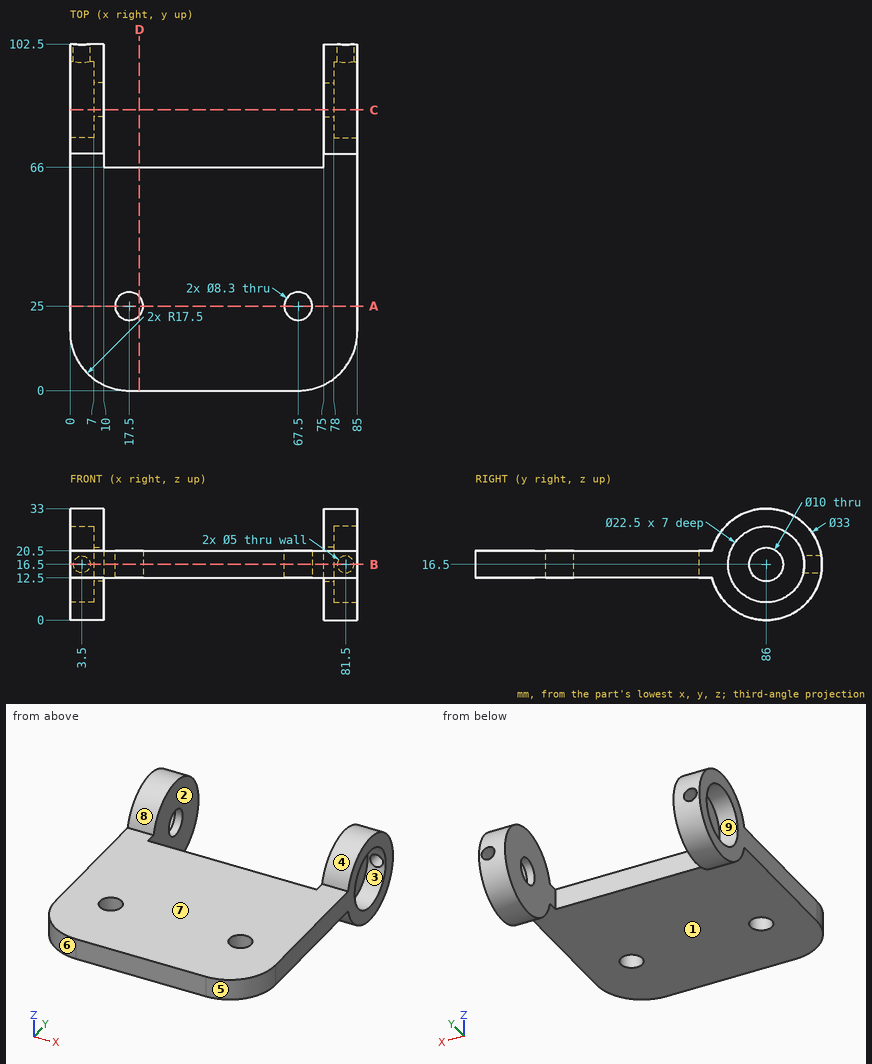
Could you check a few things on this drawing? It's one solid part, dimensions in mm from its lowest x, y, z. A direction names the side the tool comes from. Round coordinates to 2 decimals unless told otherwise and drop trailing zeros. Loops run counter-clockwise (first coordinate to the right, second up) from the corner with the lowest first, then second, coordinate; pieces in that order, holes last. Notation, with made-up numbers: M 31,-30.75 L 42,-30.75 A23 ccw 42,7.25 Z; hole C 12,48 d11. An arc over 180 degrees is marked long. Write each question's results on one line, items separated by ' | '. Start each with the question number.
(1) I want a section at D-D (x = 20.5). Please give me the cut outline in (y, z).
(2) I want a section at C-C (y = 83). Please give me the cut outline in (x, z).
(3) I want a section at B-B (z = 16.5). State how many separate pieces and enclosed holes the cut face has, then the cut area to 3 significant figures.
(4) Will these pins go through, and if not, where does the flat tip stop? P1, Ø3, axis at x = 59.5, z = 11.5, coming from the +Y side; P2, Ø16, axis at y = 86, z = 16.5, coming from the +X side; P3, Ø12, axis at x = 21, z = 28.5, coming from the +Y side; P4, Ø18, axis at y = 86, z = 16, coming from the -X side.
(5) On a 3-axis mill with a long thin cutter (end or side, diameter ignored), from which of +Z, -Z, +X, -X, +Y, -Y can I reach the whole of each face in a straight line? I mean the marked faces 1, 2, 3, 4 and 5. Say none if no direction works.
(6) Thinking about a two-plate mould opening in Z: for the marked faces 6, 7, 8 and 9, which applies, pulls with the +Z half, pulls with the -Z half, needs draft (parallel to the pull), parting line crosses it, or undercut?
(7) I want a section at A-A (y = 25). Please give me the cut outline in (x, z).
(8) If I drill on probe 1 along X at (y, z) = (99.1, 16.5); probe 2 along X at (y, z) = (80.5, 20); probe 3 along X at (y, z) = (75, 9), over which ranges is the centre line in solid material (lowest first)? Write a range as from..to.
Solved:
1) outline: M 0,12.5 L 22.13,12.5 L 22.13,20.5 L 0,20.5 Z; M 27.87,12.5 L 66,12.5 L 66,20.5 L 27.87,20.5 Z
2) outline: M 0,0.28 L 10,0.28 L 10,12.5 L 7,12.5 L 7,5.66 L 0,5.66 Z; M 0,27.34 L 7,27.34 L 7,20.5 L 10,20.5 L 10,32.72 L 0,32.72 Z; M 75,0.28 L 85,0.28 L 85,5.66 L 78,5.66 L 78,12.5 L 75,12.5 Z; M 75,20.5 L 78,20.5 L 78,27.34 L 85,27.34 L 85,32.72 L 75,32.72 Z
3) separate pieces: 5 | enclosed holes: 2 | area: 5,670 mm²
4) P1: stops at y = 66 | P2: stops at x = 78 | P3: passes through | P4: stops at x = 7
5) face 1: -Z, +X, -X, -Y | face 2: +Z, -Z, +Y | face 3: +X | face 4: +X, -X | face 5: +Z, -Z, +X, -Y
6) face 6: needs draft | face 7: pulls with the +Z half | face 8: parting line crosses it | face 9: undercut
7) outline: M 0,12.5 L 13.35,12.5 L 13.35,20.5 L 0,20.5 Z; M 21.65,12.5 L 63.35,12.5 L 63.35,20.5 L 21.65,20.5 Z; M 71.65,12.5 L 85,12.5 L 85,20.5 L 71.65,20.5 Z
8) probe 1: x = 0..1, 6..10, 75..79, 84..85 | probe 2: x = 7..10, 75..78 | probe 3: x = 0..10, 75..85
